Part model, mm, in its own coordinate system. A direction names the side the tool comes from. Round coordinates to 2 decimals unless told otherwise and drop trailing zeros. Loops run counter-clockwise (first coordinate to the right, second up) from the corner with the lowest first, then second, coordinate; pieces in that order, holes last. Notation, with made-up numbers: (-11, 68.5) - (24, 68.5) arc R31 cw to (24, 94.5) - close; hole circle Ø8 at (79.25, -24). An arc over 180 degrees is marked (long way). Write each question's results on one line, items separated by ' | '. Start each with the question number.
(1) Cut at D-D, the plane y = 16. List the corners of the cut face in (x, z).
(2) Cut at B-B, the plane y = 22. List the corners of the cut face in (x, z).
(3) Tool access for faces 1 (the face through (-8, 8, 0)), 2 (the face through (-12, 16, 8.331)): list every direction of +Z, -Z, +X, -X, +Y, -Y with a clear straight run to the whole face (end or side of a thin tool).
(4) Drill centre lines: L1, parallel to X at y = 17, z = 13; L2, parallel to Z at x = -10, y = 9.5; L3, parallel to Y at x = -8.25, z = 12.75. Where is each one in solid material? Low to high.
(5) Mould opens along Y. For faces 3 (the face through (-7.747, 18, 12)), 4 (the face through (-8, -7.823, 8)), 5 (the face through (-4.2, 12.2, 12.2)), 6 (the face through (-8, 8.052, 12)) say: released by +Y, released by -Y, zero draft, split by the parting line, or undercut.
(6) Flat gauge pins, fed straight in: P1, Ø5, axis at x = -14, z = 13.5, coming from the +Y side; P2, Ø4, axis at x = -11, y = 16, coming from the +Z side; P3, Ø4, axis at y = 18, z = 11.5, coming from the -X side. Where does each tip first touch, or does it go through?
(7) Cut at C-C, the plane x = -1. List the corners of the cut face in (y, z).
(8) Cut at A-A, the plane x = -11.5. List the corners of the cut face in (y, z), then the cut area to 3 significant figures.
from build123d import *

# Parameters (mm, degrees)
F0_W     = 15.4432
F0_H     = 16.129
F1_DEPTH = 16.3068
F2_W     = 15.875
F2_H     = 7.9756
F3_DEPTH = 7.6962
F5_DEPTH = 25.4


with BuildPart() as f1:
    # F0 (on Top) → F1 (new body)
    with BuildSketch(Plane.XY):
        Polygon((0, -7.8232), (0, 0), (0, 7.7978), (-15.4432, 7.7978), (-15.4432, -7.8232), align=None)
        with Locations((-7.7216, 15.8623)):
            Rectangle(F0_W, F0_H)
    extrude(amount=F1_DEPTH)

    # F2 (on face) → F3 (cut)
    with BuildSketch(Plane(origin=(-15.4432, 0, 0), x_dir=(0, -1, 0), z_dir=(-1, 0, 0))):
        with Locations((-15.9893, 12.319)):
            Rectangle(F2_W, F2_H)
    extrude(amount=-F3_DEPTH, mode=Mode.SUBTRACT)

    # F4 (on face) → F5 (cut)
    with BuildSketch(Plane.YZ):
        Polygon((16.4338, 16.3068), (8.0518, 16.3068), (8.0518, 8.1788), align=None)
    extrude(amount=-F5_DEPTH, mode=Mode.SUBTRACT)


solid = f1.part
A:
1) outline: (-15.44, 0) - (0, 0) - (0, 15.89) - (-7.75, 15.89) - (-7.75, 8.33) - (-15.44, 8.33) - close
2) outline: (-15.44, 0) - (0, 0) - (0, 16.31) - (-7.75, 16.31) - (-7.75, 8.33) - (-15.44, 8.33) - close
3) face 1: -Z, +X, -X, +Y, -Y | face 2: +Z, -X, +Y
4) L1: -7.75 to 0 | L2: 0 to 8.33 | L3: -7.82 to 8.05
5) face 3: zero draft | face 4: released by -Y | face 5: undercut | face 6: undercut
6) P1: y = 8.05 | P2: z = 8.33 | P3: x = -7.75
7) outline: (-7.82, 0) - (23.93, 0) - (23.93, 16.31) - (16.43, 16.31) - (8.05, 8.18) - (8.05, 16.31) - (-7.82, 16.31) - close
8) outline: (-7.82, 0) - (23.93, 0) - (23.93, 8.33) - (8.21, 8.33) - (8.05, 8.18) - (8.05, 16.31) - (-7.82, 16.31) - close | area: 391 mm2
